Input: part model. Units: mm. Frame: model coordinates. Coordinates: 2 decimals unless noted, no trailing zeros. Write each loop counter-clockwise with the first axis right and the second up, starting at its lowest first coordinate (ties: lowest second). Pieces come first, ordered by that corner, then holes. Notation, with made-up numbers: M 7,-14 L 59,-14 A23 cw 59,6 Z; hole C 55,-2.5 d2. An arc over 180 degrees is marked long. Write each question's results on one line, items separated by ' | '. Start each with the question number.
1. Section query D-D, the plane z = 366. Output: boundary loops of the cut face in (x, y).
2. Section query A-A, the plane z = 195. Output: boundary loops of the cut face in (x, y), and give its area (3 significant figures).
3. Section query B-B, the plane x = -75. Output: boundary loops of the cut face in (y, z), and give its area (3 significant figures).
4. Ray query, probe 1 along Z at (x, y) = (-5, -2.7); probe 2 along Z at (x, y) = (-30, -3.6); probe 3 along X at (y, z) = (-2.2, 375). Return the intervals inside material, ascending.
5. First-contact query: pin 1 (2.5 mm diameter, centred on y = -2, z = 375, fed in from -X); pin 2 (4 mm diameter, centred on x = -75, z = 195, fed in from +Y); pin 3 (1 mm diameter, centred on x = -25, y = -2, fed in from -Z). Flat tips, straight axial feed; report the tip coordinate or a pass-through.
6. Section query C-C, the plane x = -30. Output: boundary loops of the cut face in (y, z).
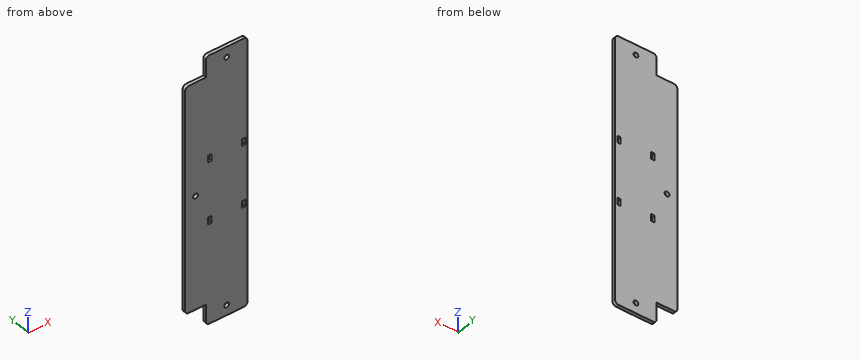
```python
from build123d import *

# Parameters (mm, degrees)
F1_W     = 5
F1_H     = 10
F1_R     = 3.5
F2_DEPTH = 4.7625


# Not quite as in the source:
# - a length typed as a fraction of an inch, garbled in the dataset ("3 / 203.2 mm" for 3/8 in), is restored


with BuildPart() as f2:
    # F1 (on Front) → F2 (new body)
    with BuildSketch(Plane.XZ):
        with BuildLine():
            ThreePointArc((-5, 0), (-1.4644660941, 1.4644660941), (0, 5))
            Line((0, 5), (0, 385))
            ThreePointArc((0, 385), (-1.4644660941, 388.5355339059), (-5, 390))
            Line((-5, 390), (-55, 390))
            ThreePointArc((-55, 390), (-58.5355339059, 388.5355339059), (-60, 385))
            Line((-60, 385), (-60, 360))
            Line((-60, 360), (-85, 360))
            ThreePointArc((-85, 360), (-88.5355339059, 358.5355339059), (-90, 355))
            Line((-90, 355), (-90, 35))
            ThreePointArc((-90, 35), (-88.5355339059, 31.4644660941), (-85, 30))
            Line((-85, 30), (-60, 30))
            Line((-60, 30), (-60, 5))
            ThreePointArc((-60, 5), (-58.5355339059, 1.4644660941), (-55, 0))
            Line((-55, 0), (-5, 0))
        make_face()
        with Locations((-54.5, 150)):
            Rectangle(F1_W, F1_H, mode=Mode.SUBTRACT)
        with Locations((-30, 15)):
            Circle(F1_R, mode=Mode.SUBTRACT)
        with Locations((-5.5, 150)):
            Rectangle(F1_W, F1_H, mode=Mode.SUBTRACT)
        with Locations((-75, 195)):
            Circle(F1_R, mode=Mode.SUBTRACT)
        with Locations((-54.5, 240)):
            Rectangle(F1_W, F1_H, mode=Mode.SUBTRACT)
        with Locations((-5.5, 240)):
            Rectangle(F1_W, F1_H, mode=Mode.SUBTRACT)
        with Locations((-30, 375)):
            Circle(F1_R, mode=Mode.SUBTRACT)
    extrude(amount=F2_DEPTH)


solid = f2.part
```
Answer:
1) outline: M -60,-4.76 L 0,-4.76 L 0,0 L -60,0 Z
2) outline: M -90,-4.76 L -78.5,-4.76 L -78.5,0 L -90,0 Z; M -71.5,-4.76 L 0,-4.76 L 0,0 L -71.5,0 Z | area: 395 mm^2
3) outline: M -4.76,30 L 0,30 L 0,191.5 L -4.76,191.5 Z; M -4.76,198.5 L 0,198.5 L 0,360 L -4.76,360 Z | area: 1,540 mm^2
4) probe 1: 0 to 145, 155 to 235, 245 to 390 | probe 2: 0 to 11.5, 18.5 to 371.5, 378.5 to 390 | probe 3: -60 to -33.5, -26.5 to 0
5) pin 1: x = -60 | pin 2: through | pin 3: z = 0
6) outline: M -4.76,0 L 0,0 L 0,11.5 L -4.76,11.5 Z; M -4.76,18.5 L 0,18.5 L 0,371.5 L -4.76,371.5 Z; M -4.76,378.5 L 0,378.5 L 0,390 L -4.76,390 Z
